from build123d import *

# Parameters (mm, degrees)
SKETCH1_W           = 10
SKETCH1_H           = 40
SKETCH1_R           = 1.65
SKETCH1_W_2         = 4.5
SKETCH1_H_2         = 12
BOSS_EXTRUDE1_DEPTH = 3


with BuildPart() as part:
    # Sketch1 → Boss-Extrude1 (new body)
    with BuildSketch(Plane(origin=(0, 0, 0), x_dir=(1, 0, 0), z_dir=(0, 1, 0))):
        with Locations((0, -15)):
            Rectangle(SKETCH1_W, SKETCH1_H)
        Circle(SKETCH1_R, mode=Mode.SUBTRACT)
        with Locations((-7.25, -1)):
            Rectangle(SKETCH1_W_2, SKETCH1_H_2)
        with Locations((7.25, -1)):
            Rectangle(SKETCH1_W_2, SKETCH1_H_2)
    extrude(amount=BOSS_EXTRUDE1_DEPTH)


solid = part.part
Work out the finished part from the listing and answer in its coordinate system (mm). A direction names the side the tool comes from. Give positions to 0.01 mm unless a question says otherwise; leave off trailing zeros. Write each loop counter-clockwise with the first axis right and the second up, starting at its lowest first coordinate (ties: lowest second). Pieces come first, ordered by that corner, then holes. Notation, with made-up numbers: (79, -22) - (116, -22) arc R22 cw to (116, -3) - close; hole circle Ø10 at (68.5, 7). An arc over 180 degrees is marked (long way). One line per item, written item: value. Start each with the question number.
1. Find section B-B (x = 0). Write down the section's boundary in (y, z).
2. Consider probe 1 along Z at (x, y) = (0, 1.6); probe 2 along X at (y, z) = (1, 0); probe 3 along X at (y, z) = (1.45, 33). Determine where each line is inside the solid, lowest interval first.
3. Find section C-C (y = 0.85). Write down the section's boundary in (x, z), then the cut area to 3 significant figures.
4. For a pull along X with two mould halves and no side action, classify faces 4 (the flat face through (0, 1, -5)), 5 (the cylindrical face through (-1.216, 1.479, -1.115)), 6 (the flat face through (9.5, 1, 1)), 7 (the flat face through (-5, 1, 21)) as +X half, -X half, draft (parallel to the pull), parting line (faces both ways), or undercut.
5. For faces 1 (the flat face through (5, 1, 21)), 2 (the flat face through (0, 0, 10)), 3 (the flat face through (-7, 1, 7)), determine the directions among +Z, -Z, +X, -X, +Y, -Y from which every point of the face is accessible in a straight line to the end or side of a thin tool.
6. Find section D-D (z = 29.5). Write down the section's boundary in (x, y).
7. Find section A-A (z = 0). Write down the section's boundary in (x, y).
Geometry results:
1. outline: (0, -5) - (3, -5) - (3, -1.65) - (0, -1.65) - close; (0, 1.65) - (3, 1.65) - (3, 35) - (0, 35) - close
2. probe 1: -5 to -1.65, 1.65 to 35
2. probe 2: -9.5 to -1.65, 1.65 to 9.5
2. probe 3: -5 to 5
3. outline: (-9.5, -5) - (9.5, -5) - (9.5, 7) - (5, 7) - (5, 35) - (-5, 35) - (-5, 7) - (-9.5, 7) - close; hole circle Ø3.3 at (0, 0)
3. area: 499 mm2
4. face 4: draft
4. face 5: undercut
4. face 6: +X half
4. face 7: -X half
5. face 1: +Z, +X, +Y, -Y
5. face 2: +Z, -Z, +X, -X, -Y
5. face 3: +Z, -X, +Y, -Y
6. outline: (-5, 0) - (5, 0) - (5, 3) - (-5, 3) - close
7. outline: (-9.5, 0) - (-1.65, 0) - (-1.65, 3) - (-9.5, 3) - close; (1.65, 0) - (9.5, 0) - (9.5, 3) - (1.65, 3) - close
